from build123d import *

# Parameters (mm, degrees)
IZIM7_W                     = 26
IZIM7_H                     = 8
Y_KSEKLIK_EKSTR_ZYON3_DEPTH = 15
IZIM8_W                     = 8
IZIM8_H                     = 26
Y_KSEKLIK_EKSTR_ZYON4_DEPTH = 4
IZIM9_W                     = 8
IZIM9_H                     = 26
Y_KSEKLIK_EKSTR_ZYON5_DEPTH = 38
IZIM11_R                    = 5
KES_EKSTR_ZYON1_DEPTH       = 44
IZIM12_R                    = 2.5
KES_EKSTR_ZYON2_DEPTH       = 44
IZIM14_R                    = 1.3
KES_EKSTR_ZYON3_DEPTH       = 4
KES_EKSTR_ZYON4_DEPTH       = 10
Y_KSEKLIK_EKSTR_ZYON6_DEPTH = 26
KES_EKSTR_ZYON5_DEPTH       = 30
Y_KSEKLIK_EKSTR_ZYON7_DEPTH = 26
Y_KSEKLIK_EKSTR_ZYON8_DEPTH = 26
KES_EKSTR_ZYON6_DEPTH       = 26


with BuildPart() as part:
    # Çizim1 → Döndür5 (revolve)
    with BuildSketch(Plane.XY, mode=Mode.PRIVATE) as d_nd_r5_sk:
        Polygon((49, 4), (60.625, 4), (60.625, 0), (45, 0), (45, 56), (49, 56), align=None)
    revolve(d_nd_r5_sk.sketch.rotate(Axis((0, 14.385693044, 0), (0, -1, 0)), 90), axis=Axis((0, 14.385693044, 0), (0, -1, 0)))

    # Çizim7 → Yükseklik-Ekstrüzyon3 (add)
    with BuildSketch(Plane.ZY.offset(-45)):
        with Locations((0, 34)):
            Rectangle(IZIM7_W, IZIM7_H)
    extrude(amount=Y_KSEKLIK_EKSTR_ZYON3_DEPTH)

    # Çizim8 → Yükseklik-Ekstrüzyon4 (add)
    with BuildSketch(Plane(origin=(0, 0, 0), x_dir=(1, 0, 0), z_dir=(0, 1, 0))):
        with Locations((-15.25, 0)):
            Rectangle(IZIM8_W, IZIM8_H)
        with BuildLine():
            Line((-11.25, 13), (-29.4469535, 34.027590711))
            ThreePointArc((-29.4469535, 34.027590711), (-45, 0), (-29.4469535, -34.027590711))
            Line((-29.4469535, -34.027590711), (-11.25, -13))
            Line((-11.25, -13), (-19.25, -13))
            Line((-19.25, -13), (-19.25, 13))
            Line((-19.25, 13), (-11.25, 13))
        make_face()
        with BuildLine():
            ThreePointArc((-29.4469535, 22.402609883), (-36.999521245, 0.188222241), (-29.673354544, -22.101855807))
            Line((-29.673354544, -22.101855807), (-24.25, -15.834868333))
            Line((-24.25, -15.834868333), (-24.25, 15.394791201))
            Line((-24.25, 15.394791201), (-29.4469535, 22.402609883))
        make_face(mode=Mode.SUBTRACT)
    extrude(amount=Y_KSEKLIK_EKSTR_ZYON4_DEPTH)

    # Çizim9 → Yükseklik-Ekstrüzyon5 (add)
    with BuildSketch(Plane(origin=(0, 0, 0), x_dir=(1, 0, 0), z_dir=(0, 1, 0))):
        with Locations((-15.25, 0)):
            Rectangle(IZIM9_W, IZIM9_H)
    extrude(amount=Y_KSEKLIK_EKSTR_ZYON5_DEPTH)

    # Çizim11 → Kes-Ekstrüzyon1 (cut)
    with BuildSketch(Plane.ZY.offset(19.25)):
        with Locations(Location((0, 14, 0), (0, 0, 180))):
            Circle(IZIM11_R)
    extrude(amount=KES_EKSTR_ZYON1_DEPTH, mode=Mode.SUBTRACT)

    # Çizim12 → Kes-Ekstrüzyon2 (cut)
    with BuildSketch(Plane(origin=(0, 0, 0), x_dir=(1, 0, 0), z_dir=(0, 1, 0))):
        with Locations(Location((-38.756522677, 38.756522677, 0), (0, 0, 270))):
            Circle(IZIM12_R)
        with Locations(Location((38.756522677, 38.756522677, 0), (0, 0, 270))):
            Circle(IZIM12_R)
        with Locations(Location((-38.756522677, -38.756522677, 0), (0, 0, 270))):
            Circle(IZIM12_R)
        with Locations(Location((38.756522677, -38.756522677, 0), (0, 0, 270))):
            Circle(IZIM12_R)
    extrude(amount=KES_EKSTR_ZYON2_DEPTH, mode=Mode.SUBTRACT)

    # Çizim14 → Kes-Ekstrüzyon3 (cut)
    with BuildSketch(Plane(origin=(0, 38, 0), x_dir=(1, 0, 0), z_dir=(0, 1, 0))):
        with Locations(Location((-13.75, 5, 0), (0, 0, 270))):
            Circle(IZIM14_R)
        with Locations(Location((-13.75, -5, 0), (0, 0, 270))):
            Circle(IZIM14_R)
        with Locations(Location((34.25, -5, 0), (0, 0, 270))):
            Circle(IZIM14_R)
        with Locations(Location((34.25, 5, 0), (0, 0, 270))):
            Circle(IZIM14_R)
    extrude(amount=-KES_EKSTR_ZYON3_DEPTH, mode=Mode.SUBTRACT)

    # Çizim15 → Kes-Ekstrüzyon4 (cut)
    with BuildSketch(Plane.ZY.offset(19.25)):
        Polygon((13, 30.072092804), (-5.072092804, 12), (13, 12), align=None)
    extrude(amount=-KES_EKSTR_ZYON4_DEPTH, mode=Mode.SUBTRACT)

    # Çizim16 → Yükseklik-Ekstrüzyon6 (add)
    with BuildSketch(Plane.XY.offset(13)):
        Polygon((30, 30), (45.409856654, 14.590143346), (45.409856654, 30), align=None)
    extrude(amount=-Y_KSEKLIK_EKSTR_ZYON6_DEPTH)

    # Çizim17 → Kes-Ekstrüzyon5 (cut)
    with BuildSketch(Plane(origin=(0, 0, 0), x_dir=(1, 0, 0), z_dir=(0, 1, 0))):
        with BuildLine():
            Line((0, -45), (0, 45))
            ThreePointArc((0, 45), (45, 0), (0, -45))
        make_face()
    extrude(amount=KES_EKSTR_ZYON5_DEPTH, mode=Mode.SUBTRACT)

    # Çizim18 → Yükseklik-Ekstrüzyon7 (add)
    with BuildSketch(Plane.XY.offset(13)):
        Polygon((43.081318457, 30), (30, 30), (45, 15), (47.625193475, 15), (47.625193475, 30), align=None)
    extrude(amount=-Y_KSEKLIK_EKSTR_ZYON7_DEPTH)

    # Çizim19 → Yükseklik-Ekstrüzyon8 (add)
    with BuildSketch(Plane.XY.offset(13)):
        Polygon((30, 30), (45, 7.621420501), (46.501965359, 7.621420501), (46.501965359, 30), align=None)
    extrude(amount=-Y_KSEKLIK_EKSTR_ZYON8_DEPTH)

    # Çizim20 → Kes-Ekstrüzyon6 (cut)
    with BuildSketch(Plane.ZY.offset(19.25)):
        Polygon((13, 33), (-5.072092804, 12), (13, 12), align=None)
    extrude(amount=-KES_EKSTR_ZYON6_DEPTH, mode=Mode.SUBTRACT)


solid = part.part
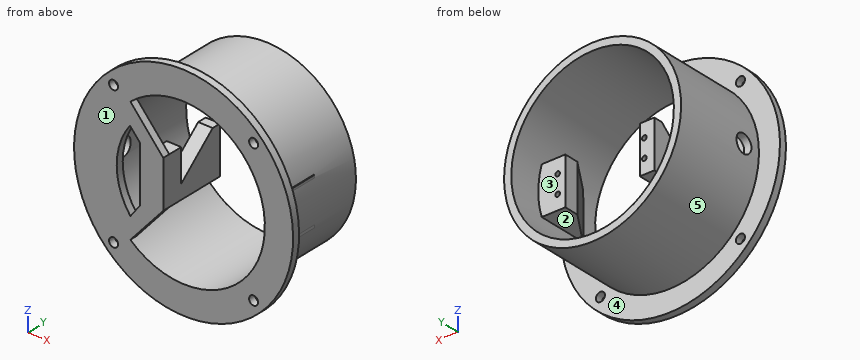
Work out the finished part from the listing and answer in its coordinate system (mm). Face numbers are marked on the shaded views. A direction names the side the tool comes from. Coordinates: 2 decimals unless noted, no trailing zeros. Order: outer loops, then holes, each group sorted by start corner. A loop starts at its lowest first (then second) coordinate and runs counter-clockwise, first axis right, second up. Notation, with made-up numbers: (-34, -6) - (-11, -6) arc R11 cw to (-11, 2) - close; hole circle Ø8 at (1, 23). An arc over 180 degrees is marked (long way). Put each result on its own line as item: value. Start each with the question number.
1) Find section D-D (z = -30). Give the vertices of the cut face in (x, y), plus the area to 3 significant figures.
2) For a pull along Z with two mould halves and no side action, classify the marked faces 3, 4 and 5 as released by +Z, released by -Z, zero draft, split by the parting line, or undercut.
3) Find section B-B (z = 0). State how many separate pieces and enclosed holes the cut face has, plus the area to 3 significant figures.
4) Find section C-C (y = 6). Give the vertices of the cut face in (x, z).
5) Flat-ended cylindrical pins translate along their axes: pin 1 (9 mm diameter, centred on x = -17, y = 25.5, fed in from -Z); pin 2 (9 mm diameter, centred on x = -17, z = -1, fed in from +Y); pin 3 (8 mm diameter, centred on y = 23.5, z = -7, fed in from +X); pin 4 (4 mm diameter, centred on x = 16.5, z = 39.5, fed in from -Y). Find the tip coordinate at first contact, or state that the pin passes through.
6) Find section A-A (x = -21.5). Give the vertices of the cut face in (y, z), plus the area to 3 significant figures.
7) Find the intervals of material crossed by line 1 (X direction, y = 36, z = -3.5); line 2 (X direction, y = 35.6, z = 5); line 3 (X direction, y = 3.5, z = -21), in increasing order. Write a range as from..to.
8) For the marked faces 1 and 2, determine the directions among +Z, -Z, +X, -X, +Y, -Y from which every point of the face is accessible in a straight line to the end or side of a thin tool.
Results list:
1. outline: (-52.68, 0) - (-25.96, 0) - (-25.96, 4) - (-33.54, 4) - (-33.54, 56) - (-38.74, 56) - (-38.74, 4) - (-52.68, 4) - close; (33.54, 0) - (52.68, 0) - (52.68, 4) - (38.74, 4) - (38.74, 56) - (33.54, 56) - close
1. area: 724 mm^2
2. face 3: undercut
2. face 4: zero draft
2. face 5: split by the parting line
3. separate pieces: 5
3. enclosed holes: 0
3. area: 1,100 mm^2
4. outline: circle Ø98 at (0, 0); (-19.25, -13) - (-11.25, -13) - (-11.25, 13) - (-19.25, 13) - close; hole circle Ø90 at (0, 0)
5. pin 1: stops at z = -47.38
5. pin 2: stops at y = 38
5. pin 3: stops at x = 48.91
5. pin 4: passes through
6. outline: (0, -56.68) - (4, -56.68) - (4, -44.03) - (56, -44.03) - (56, -39.53) - (0, -39.53) - close; (0, -24.84) - (4, -24.84) - (4, 24.84) - (0, 24.84) - close; (0, 39.53) - (56, 39.53) - (56, 44.03) - (4, 44.03) - (4, 56.68) - (0, 56.68) - close
6. area: 804 mm^2
7. line 1: x = -48.87..-44.86, -19.25..-11.25, 30..48.87
7. line 2: x = -48.74..-44.72, -19.25..-15.05, -12.45..-11.25, 30..32.95, 35.55..48.74
7. line 3: x = -56.87..-30.46, -28.41..-18.17, 39.8..56.87
8. face 1: +Z, -Z, +X, -X, -Y
8. face 2: +Y, -Y
